Answer from the drawing. Dimensions are ordinates in mm from the lowest x, y and z of the part. A direction names the side the tool comes from. Round coordinates to 2 decimals unless told otherwise and drop trailing zeros. Loops run counter-clockwise (first coordinate to the right, second up) from the corner with the lowest first, then second, coordinate; pieces in that order, holes last. Notation, with made-up numbers: (74, -3) - (78, -3) arc R20 cw to (78, 35) - close; hole circle Ø3 at (66.25, 55). An arc over 180 degrees is marked (long way). Return JSON: item names as keys, results as strings.
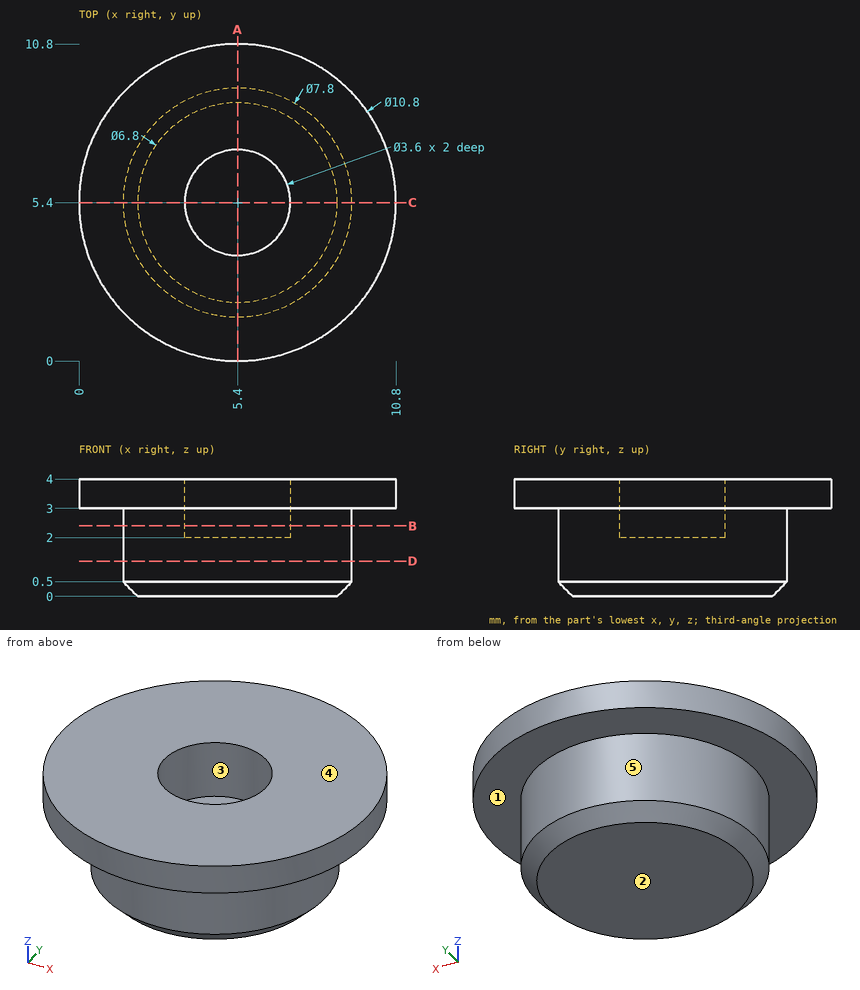
1) A tool of negligible diameter and unlimited length cuts with its end or side. For the marked faces 1 and 2, from which of +Z, -Z, +X, -X, +Y, -Y can it reach the whole face along a straight path? Write none if from no direction.
Verdict:
{"face 1": "-Z", "face 2": "-Z, +X, -X, +Y, -Y"}
2) Section B-B (z = 2.4) is taken. Give the vertices of the cut face in (x, y).
Verdict:
{"outline": "circle Ø7.8 at (5.4, 5.4); hole circle Ø3.6 at (5.4, 5.4)"}
3) Determine the mould class of the marked faces 3, 4 and 5 for opening direction Y: pulls with the +Y half, pulls with the -Y half, needs draft (parallel to the pull), parting line crosses it, or undercut.
Verdict:
{"face 3": "undercut", "face 4": "needs draft", "face 5": "parting line crosses it"}
4) Section A-A (x = 5.4) is taken. Give the vertices of the cut face in (y, z), and give its area (4 significant figures).
Verdict:
{"outline": "(0, 3) - (1.5, 3) - (1.5, 0.5) - (2, 0) - (8.8, 0) - (9.3, 0.5) - (9.3, 3) - (10.8, 3) - (10.8, 4) - (7.2, 4) - (7.2, 2) - (3.6, 2) - (3.6, 4) - (0, 4) - close", "area": "26.75 mm2"}
5) Flat-ended cylindrical pins translate along their axes: pin 1 (1.1 mm diameter, centred on x = 6, y = 5.5, fed in from +Z); pin 2 (3 mm diameter, centred on x = 3.5, y = 6.5, fed in from -Z); pin 3 (1.5 mm diameter, centred on y = 1.5, z = 1, fed in from +X). Find the tip coordinate at first contact, or state that the pin passes through.
Verdict:
{"pin 1": "stops at z = 2", "pin 2": "stops at z = 0", "pin 3": "stops at x = 7.7"}
6) Section D-D (z = 1.2) is taken. Give the vertices of the cut face in (x, y), and give its area (3 significant figures).
Verdict:
{"outline": "circle Ø7.8 at (5.4, 5.4)", "area": "47.8 mm2"}
7) Find the intervals of material crossed by L1, parallel to Y at x = 5.4, z = 3.4; L2, parallel to Y at x = 5.4, z = 2.7; L3, parallel to Z at x = 4.75, y = 1, in increasing order.
Verdict:
{"L1": "y = 0 to 3.6, 7.2 to 10.8", "L2": "y = 1.5 to 3.6, 7.2 to 9.3", "L3": "z = 3 to 4"}
